Drawing for the job (mm, zero at the part's lowest x, y, z). Round coordinates to 2 decimals unless told otherwise and drop trailing zeros. Order: outer loops, then holes, each group sorted by start corner. A loop starts at its lowest first (then second) coordinate and runs counter-clockwise, first axis right, second up. Notation, with made-up numbers: (-21, 17) - (3, 17) arc R21 ccw to (3, 31) - close; hole circle Ø4 at (33, 9). An arc over 180 degrees is marked (long way). Put each result on its own line as item: value. Start each with the question number.
Item 1: Pin check, flat tip, straight feed: pin 1 Ø0.6 at (x, y) = (29.5, 0.5) entering from -Z. Stop position of the tip, or through.
Item 2: Probe probe 1 along X at (y, z) = (1.3, 49.5); probe 2 along Z at (x, y) = (39, 1.4). List the from-to ranges inside material, lowest first.
Item 3: Saw through at A-A on z = 3. List the corners of the cut face in (x, y).
Item 4: Saw through at B-B on x = 32. List the corners of the cut face in (y, z).
Item 5: Saw through at C-C on y = 0.4. State how many separate pieces and enclosed holes the cut face has, plus the area to 3 significant figures.
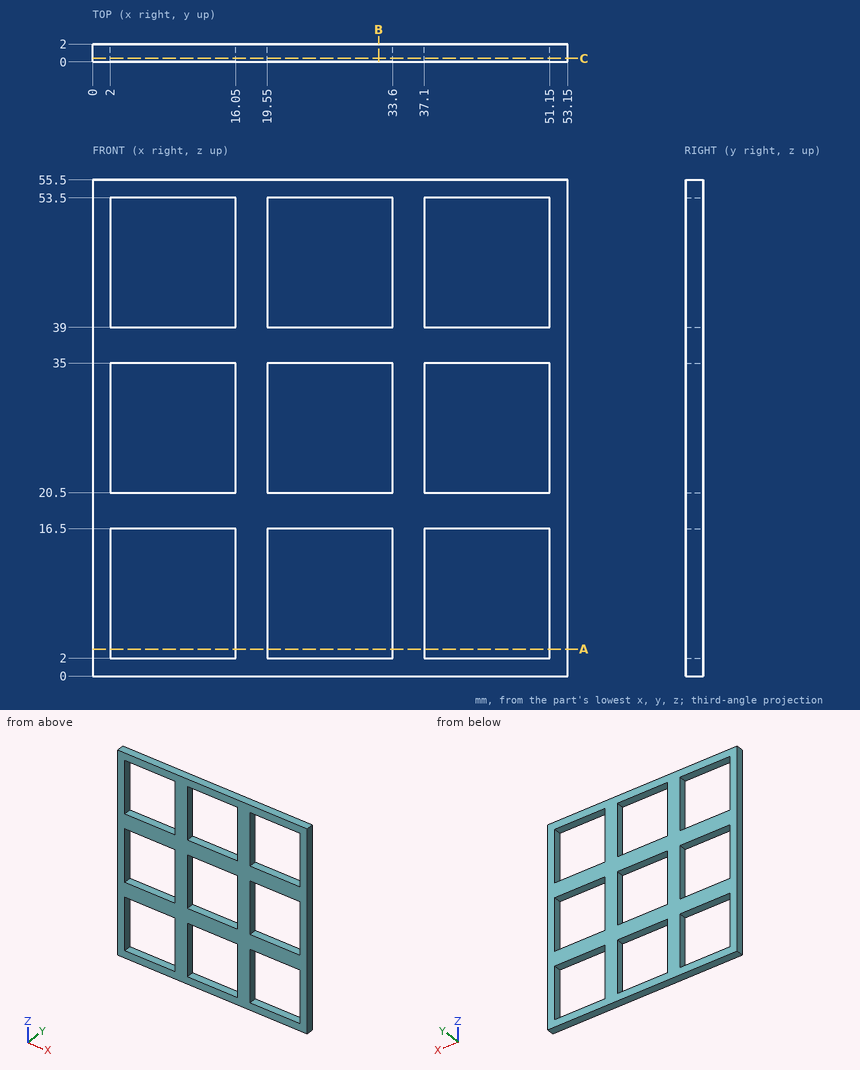
Results found:
1. pin 1: stops at z = 0
2. probe 1: x = 0 to 2, 16.05 to 19.55, 33.6 to 37.1, 51.15 to 53.15
2. probe 2: z = 0 to 2, 16.5 to 20.5, 35 to 39, 53.5 to 55.5
3. outline: (0, 0) - (2, 0) - (2, 2) - (0, 2) - close; (16.05, 0) - (19.55, 0) - (19.55, 2) - (16.05, 2) - close; (33.6, 0) - (37.1, 0) - (37.1, 2) - (33.6, 2) - close; (51.15, 0) - (53.15, 0) - (53.15, 2) - (51.15, 2) - close
4. outline: (0, 0) - (2, 0) - (2, 2) - (0, 2) - close; (0, 16.5) - (2, 16.5) - (2, 20.5) - (0, 20.5) - close; (0, 35) - (2, 35) - (2, 39) - (0, 39) - close; (0, 53.5) - (2, 53.5) - (2, 55.5) - (0, 55.5) - close
5. separate pieces: 1
5. enclosed holes: 9
5. area: 1,120 mm²
